For this review, take the finished solid that the model builds, in its own axes (mm). Face numbers are marked on the shaded views. A direction names the side the tool comes from. Round coordinates to 2 decimals unless told otherwise and drop trailing zeros. Loops run counter-clockwise (first coordinate to the right, second up) from the corner with the lowest first, then second, coordinate; pieces in that order, holes last.
1) Take a section at A-A (z = 114.3). State the section outline as (x, y) points, then the cut area to 3 significant figures.
2) Tool access review of the marked faces 1 and 2: name each direction out of +Z, -Z, +X, -X, +Y, -Y from which nothing blocks a thin tool from reaching the whole face with its end or side.
3) Wall thickness on L1, parallel to Y at x = -3, z = 114; L2, parallel to Z at x = 34, y = -137.5; L3, parallel to X at y = -130, z = 103.5: over which ranges is each line inside the solid? List them lowest first.
4) Take a section at C-C (y = -61). State the section outline as (x, z) points.
5) Take a section at B-B (y = -114.3). State the section outline as (x, z) points.
6) Take a section at D-D (z = 79.5). State the section outline as (x, y) points.
7) Insertion check: pin 1 (7.5 mm diameter, centred on x = 92.32, y = -114.3, fed in from +Z); pin 2 (12 mm diameter, centred on x = 70.5, y = -111.5, fed in from +Z). Each pin has a flat end and moves straight along its axis. Give the tip position at first contact, or say it passes through.
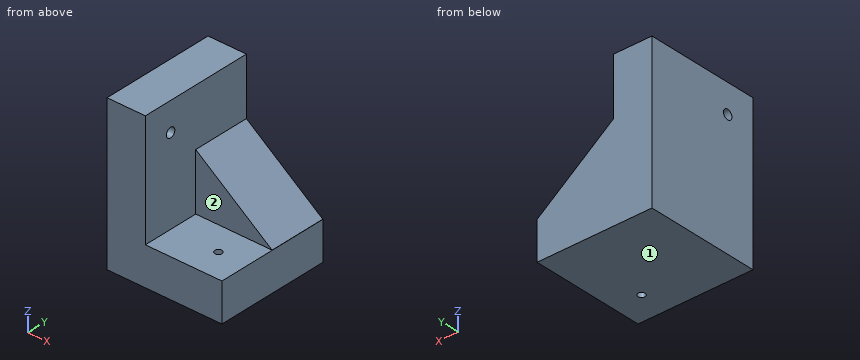
```python
from build123d import *

# Parameters (mm, degrees)
F1_DEPTH = 152.4
F2_W     = 101.356273
F2_H     = 76.407738
F3_DEPTH = 76.2
F5_DEPTH = 84.108479
F7_D     = 9.525
F9_D     = 12.7


with BuildPart() as f1:
    # F0 (on Front) → F1 (new body)
    with BuildSketch(Plane.XZ):
        Polygon((28.823013, 0), (28.823013, 152.4), (-21.976987, 152.4), (-21.976987, -50.8), (130.423013, -50.8), (130.423013, 0), align=None)
    extrude(amount=F1_DEPTH)

    # F2 (on face) → F3 (join)
    with BuildSketch(Plane.XY):
        with Locations((79.501149, -38.203869)):
            Rectangle(F2_W, F2_H)
    extrude(amount=F3_DEPTH)

    # F4 (on face) → F5 (cut)
    with BuildSketch(Plane.XZ.offset(76.407738)):
        Polygon((130.179286, 76.2), (28.823013, 76.2), (130.179286, 0), align=None)
    extrude(amount=-F5_DEPTH, mode=Mode.SUBTRACT)

    # F7 (through all)
    with Locations(Plane.XY):
        with Locations((92.323013, -114.3)):
            Hole(F7_D / 2)

    # F9 (through all)
    with Locations(Plane.YZ.offset(28.823013)):
        with Locations((-114.3, 114.3)):
            Hole(F9_D / 2)


solid = f1.part
```
Response:
1. outline: (-21.98, -152.4) - (28.82, -152.4) - (28.82, -120.65) - (-21.98, -120.65) - close; (-21.98, -107.95) - (28.82, -107.95) - (28.82, 0) - (-21.98, 0) - close
1. area: 7,100 mm2
2. face 1: -Z, +X, -X, +Y, -Y
2. face 2: +Z, +X, -Y
3. L1: y = -152.4 to -120.64, -107.96 to 0
3. L2: z = -50.8 to 0
3. L3: x = -21.98 to 28.82
4. outline: (-21.98, -50.8) - (130.42, -50.8) - (130.42, 0) - (130.18, 0) - (28.82, 76.2) - (28.82, 152.4) - (-21.98, 152.4) - close
5. outline: (-21.98, -50.8) - (87.56, -50.8) - (87.56, 0) - (28.82, 0) - (28.82, 107.95) - (-21.98, 107.95) - close; (-21.98, 120.65) - (28.82, 120.65) - (28.82, 152.4) - (-21.98, 152.4) - close; (97.09, -50.8) - (130.42, -50.8) - (130.42, 0) - (97.09, 0) - close
6. outline: (-21.98, -152.4) - (28.82, -152.4) - (28.82, 0) - (-21.98, 0) - close
7. pin 1: passes through
7. pin 2: stops at z = 0
